Part print with two shaded views. Sizes in mm from the minimum x, y, z corner. A direction names the side the tool comes from. Coordinates: 2 decimals unless noted, no trailing zeros. Loops run counter-clockwise (first coordinate to the right, second up) from the corner with the lowest first, then second, coordinate; pieces in that order, holes last. Notation, with made-up numbers: (17.5, -22) -> (63.5, -22) arc R13 cw to (63.5, 1) -> close; hole circle Ø1 at (38, 49.5). An arc over 180 degrees is marked (long way). Write each question's results on one line, items separated by ' | '.
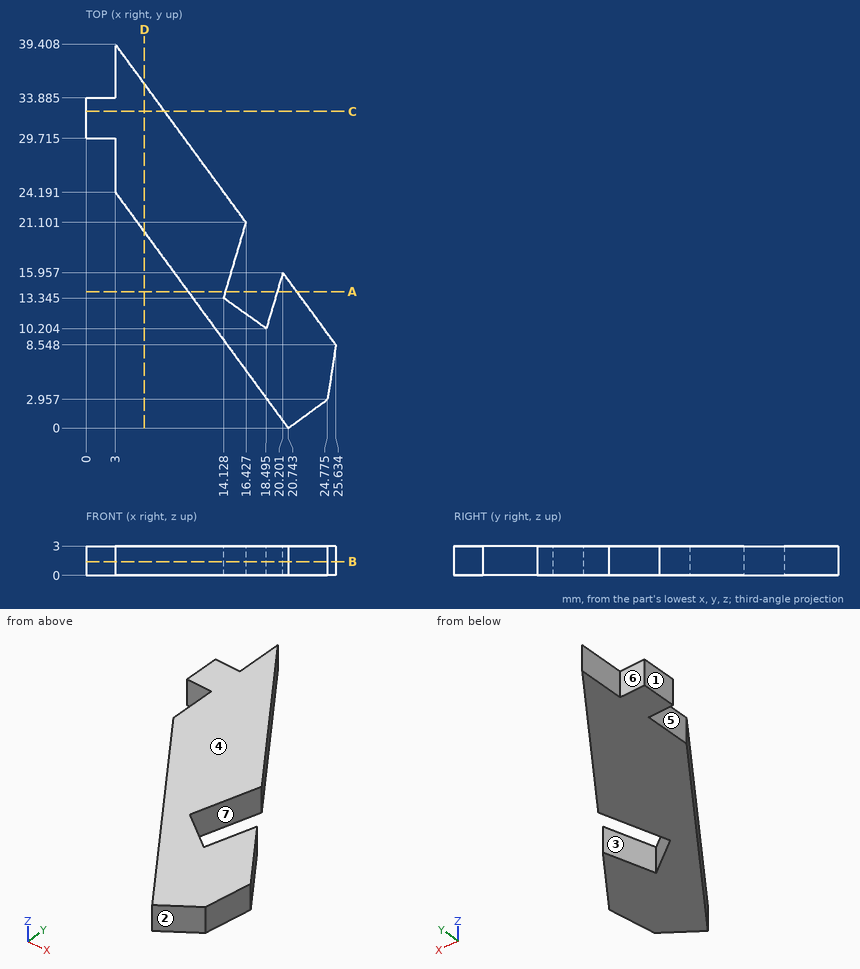
Q1. Drop flat-ended pins along their axis: pin 1 (1.5 mm diameter, centred on x = 1.5, z = 1.5, fed in from +Y) (1 decimal); pin 2 (1 mm diameter, centred on x = 16, z = 2.5, fed in from +Y) (1 decimal); pin 3 (1.5 mm diameter, centred on x = 16, z = 1, fed in from -Y) (1 decimal). Give the stop position or say it passes through.
Results are:
pin 1: y = 33.9 | pin 2: y = 22.4 | pin 3: y = 5.4
Q2. Which spindle directions (+Z, -Z, +X, -X, +Y, -Y) get a long thin tool onto all of the face, cutting with end or side? Do the marked faces 5, 6 and 7. Say none if no direction does.
Results are:
face 5: +Z, -Z, -X, -Y | face 6: +Z, -Z, -X, +Y | face 7: +Z, -Z
Q3. Cut at A-A on y = 14. Write the cut outline in (x, z) (1 decimal).
Results are:
outline: (10.5, 0) -> (14.3, 0) -> (14.3, 3) -> (10.5, 3) -> close; (19.6, 0) -> (21.6, 0) -> (21.6, 3) -> (19.6, 3) -> close
Q4. Cut at B-B on z = 1.4. Write the cut outline in (x, y) (1 decimal), and give its area (3 significant figures).
Results are:
outline: (0, 29.7) -> (3, 29.7) -> (3, 24.2) -> (20.7, 0) -> (24.8, 3) -> (25.6, 8.5) -> (20.2, 16) -> (18.5, 10.2) -> (14.1, 13.3) -> (16.4, 21.1) -> (3, 39.4) -> (3, 33.9) -> (0, 33.9) -> close | area: 294 mm^2
Q5. Cut at C-C on y = 32.5. Write the cut outline in (x, z), and give its area (3 significant figures).
Results are:
outline: (0, 0) -> (8.07, 0) -> (8.07, 3) -> (0, 3) -> close | area: 24.2 mm^2
Q6. Wall check: L1, parallel to X at y = 13, z = 0.7 (1 decimal); L2, parallel to X at y = 6.5, z = 1.55 (1 decimal); L3, parallel to X at y = 7, z = 0.75 (1 decimal). Give the ranges that are in metal, low to high. Write a range as from..to.
Results are:
L1: 11.2..14.6, 19.3..22.4 | L2: 16..25.3 | L3: 15.6..25.4
Q7. Cut at D-D on x = 6. Write the cut outline in (y, z).
Results are:
outline: (20.1, 0) -> (35.32, 0) -> (35.32, 3) -> (20.1, 3) -> close
Q8. Pull direction X, two halves, no side cores. Call the marked faces 1, 2, 3 and 4: +X half, -X half, draft (parallel to the pull), parting line (faces both ways), or undercut.
Results are:
face 1: -X half | face 2: +X half | face 3: undercut | face 4: draft
